Input: part model. Units: mm. Frame: model coordinates. Face numbers are marked on the shaded views. A direction names the side the tool comes from. Give positions to 0.01 mm unless a question says otherwise; leave off trailing zeros. Loops run counter-clockwise (first coordinate to the right, second up) from the corner with the lowest first, then second, coordinate; pieces in that order, holes last. Notation, with made-up numbers: M 33.5,-38.5 L 47.5,-38.5 A38 cw 47.5,-0.5 Z; hole C -7.5,-30.5 d3. An arc over 180 degrees is marked long. Use a Markdown table: item, result. Add a question column.
from build123d import *

# Parameters (mm, degrees)
CHAMFER2_SIZE      = 0.5
CUT_EXTRUDE1_DEPTH = 2


with BuildPart() as part:
    # Sketch1 → Revolve1 (revolve)
    with BuildSketch(Plane.XY):
        Polygon((0, 3), (65, 3), (65, 1.5), (67, 1.5), (67, 2), (72, 2), (72, 0), (-4, 0), (-4, 4.5), (0, 4.5), align=None)
    revolve(axis=Axis((-15.448246648, 0, 0), (1, 0, 0)))

    # Chamfer2
    chamfer2_edges = [part.edges().sort_by_distance(p)[0] for p in [
        (-4, -4.5, 0),
    ]]
    chamfer(chamfer2_edges, length=CHAMFER2_SIZE)

    # Sketch2 → Cut-Extrude1 (cut)
    with BuildSketch(Plane.ZY.offset(4)):
        Polygon((0, 1.732050808), (-1.5, 0.866025404), (-1.5, -0.866025404), (0, -1.732050808), (1.5, -0.866025404), (1.5, 0.866025404), align=None)
    extrude(amount=-CUT_EXTRUDE1_DEPTH, mode=Mode.SUBTRACT)


solid = part.part
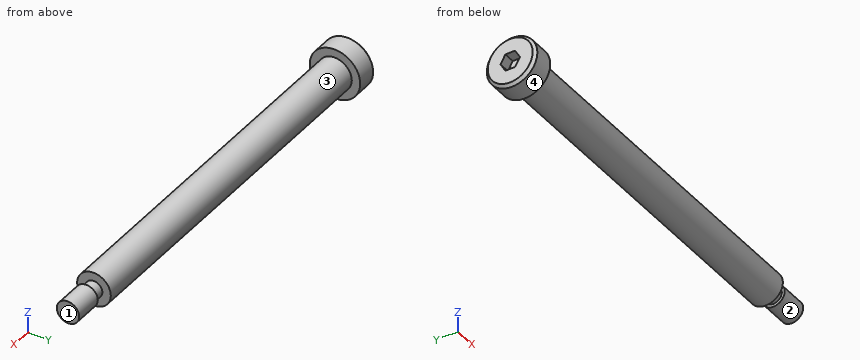
1) Ray query, line 1 (X direction, y = -2.5, z = -1.5); line 2 (X direction, y = -3.5, z = -0.5); line 3 (X direction, y = -1.25, z = -1.5). Return the intervals inside material, ascending. Write a range as [from, to].
2) Contact query for flat-ended pins moving along their axis: P1, Ø1.5, axis at x = 11.5, z = -2, coming from the -Y side; P2, Ø5, axis at x = 23.5, y = 1, coming from the -Z side; P3, Ø2, axis at x = 25, z = -2, coming from the -Y side. Output: stop coordinate, or through.
3) Pull-direction query (Z, two-part tool) for the marked faces 1 and 2; classes: pulls with the +Z half, pulls with the -Z half, needs draft (parallel to the pull), parting line crosses it, or undercut.
4) Reachability of the marked faces 3 and 4 from +Z, -Z, +X, -X, +Y, -Y: full face, straight path, thin tool, end or side. Return the list, or none.
5) Section query A-A, the plane y = 0. Return the cut outline in (x, z), and give its area (3 significant figures).
6) Section query B-B, the plane x = 21. Return the cut outline in (y, z), and give its area (3 significant figures).
Entries:
| question | item | result |
|---|---|---|
| 1 | line 1 | x = [-4, 65] |
| 1 | line 2 | x = [-4, 0] |
| 1 | line 3 | x = [-4, 65], [67, 72] |
| 2 | P1 | stops at y = -2.73 |
| 2 | P2 | stops at z = -3 |
| 2 | P3 | stops at y = -2.83 |
| 3 | face 1 | needs draft |
| 3 | face 2 | parting line crosses it |
| 4 | face 3 | +X |
| 4 | face 4 | +X, -X |
| 5 | outline | M -4,-4 L -3.5,-4.5 L 0,-4.5 L 0,-3 L 65,-3 L 65,-1.5 L 67,-1.5 L 67,-2 L 72,-2 L 72,2 L 67,2 L 67,1.5 L 65,1.5 L 65,3 L 0,3 L 0,4.5 L -3.5,4.5 L -4,4 L -4,1.5 L -2,1.5 L -2,-1.5 L -4,-1.5 Z |
| 5 | area | 446 mm² |
| 6 | outline | C 0,0 d6 |
| 6 | area | 28.3 mm² |
